Source: CAD feature listing. Evaluate the final solid. Frame: model axes, mm. Face numbers are marked on the shaded views. A direction names the side the tool comes from. Give positions to 0.01 mm unless a question says otherwise; leave off trailing zeros. Order: outer loops, then holes, each group sorted by start corner. A loop starts at its lowest first (then second) coordinate and runs counter-clockwise, first axis right, second up. Notation, with made-up numbers: M 86.5,40 L 121.5,40 A22 cw 121.5,69 Z; hole C 53.25,36.25 d6. An arc over 180 degrees is marked long. Answer as a JSON object with one key per item and string values. Group by question number.
1. Material intervals for L1, parallel to X at y = -12.5, z = -7 (3 decimals); L2, parallel to Z at x = 4, y = 0 (1 decimal); L3, parallel to Z at x = -0.5, y = 0, sorted ascending. Write a range as [from, to].
2. Pin query (flat end, axial travel): P1, Ø4, axis at x = 1.5, y = -1.5, coming from the -Z side; P2, Ø6, axis at x = -4, z = 8.5, coming from the -Y side; P3, Ø3, axis at x = -1, y = -6.5, coming from the +Z side. Return the tip coordinate at first contact, or that it passes through.
3. Pull-direction query (Y, two-part tool) for the marked faces 1, 2, 3 and 4; classes: +Y half, -Y half, draft (parallel to the pull), parting line (faces both ways), or undercut.
4. Section query D-D (z = -11.5). Output: boundary loops of the cut face in (x, y) (3 decimals).
5. Set-up query: the marked faces 5 and 6. Return all of +Z, -Z, +X, -X, +Y, -Y with unobstructed straight access to the full face (end or side cutting, diameter ignored); none if empty.
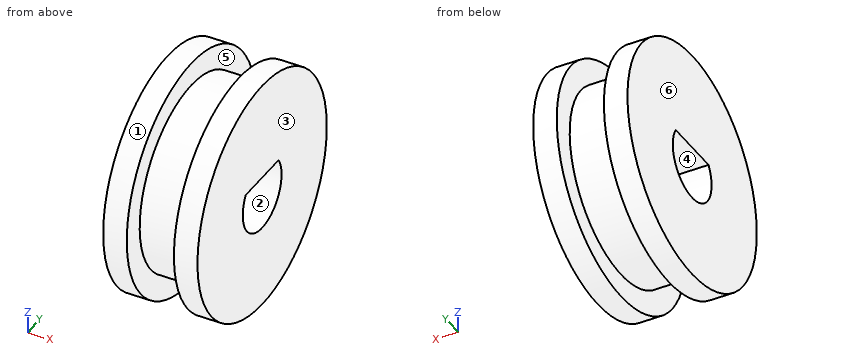
from build123d import *

# Parameters (mm, degrees)
F3_DEPTH      = 6.35
F3_DEPTH_BACK = 6.35


with BuildPart() as f1:
    # F0 (on Front) → F1 (revolve)
    with BuildSketch(Plane.XZ):
        Polygon((-6.35, 15.875), (-6.35, 4.7625), (6.35, 4.7625), (6.35, 15.875), (3.175, 15.875), (3.175, 12.7), (-3.175, 12.7), (-3.175, 15.875), align=None)
    revolve(axis=Axis((0, 0, 0), (1, 0, 0)))

    # F2 (on Right) → F3 (join, two sides)
    with BuildSketch(Plane.YZ) as f3_sk:
        with BuildLine():
            Line((-4.0286233691, 2.54), (4.0286233691, 2.54))
            ThreePointArc((4.0286233691, 2.54), (0, 4.7625), (-4.0286233691, 2.54))
        make_face()
    extrude(amount=F3_DEPTH)
    extrude(f3_sk.sketch, amount=-F3_DEPTH_BACK)


solid = f1.part
Answer sheet:
{
 "1": {"L1": "[-6.35, -3.175], [3.175, 6.35]", "L2": "[-15.9, -4.8], [2.5, 15.9]", "L3": "[-12.7, -4.76], [2.54, 12.7]"},
 "2": {"P1": "z = -15.87", "P2": "y = -14.89", "P3": "z = 11.67"},
 "3": {"face 1": "parting line", "face 2": "undercut", "face 3": "draft", "face 4": "undercut"},
 "4": {"outline": "M -6.35,-10.944 L -3.175,-10.944 L -3.175,-5.389 L 3.175,-5.389 L 3.175,-10.944 L 6.35,-10.944 L 6.35,10.944 L 3.175,10.944 L 3.175,5.389 L -3.175,5.389 L -3.175,10.944 L -6.35,10.944 Z"},
 "5": {"face 5": "none", "face 6": "+Z, -Z, -X, +Y, -Y"}
}
